Input: part model. Units: mm. Frame: model coordinates. Face numbers are marked on the shaded views. A direction names the side the tool comes from. Coordinates: 2 decimals unless noted, no trailing zeros. Write each loop counter-clockwise with the first axis right and the second up, starting at its lowest first coordinate (ties: lowest second). Pieces come first, ordered by that corner, then holes.
from build123d import *

# Parameters (mm, degrees)
F0_W      = 96
F0_H      = 12
F1_DEPTH  = 18
F3_DEPTH  = 10
F4_R      = 17
F5_R      = 6
F6_DEPTH  = 10.001
F7_W      = 14
F7_H      = 15
F8_DEPTH  = 25
F9_R      = 7
F10_DEPTH = 25
F11_R     = 5
F12_DEPTH = 12.001


with BuildPart() as f1:
    # F0 (on Front) → F1 (new body, symmetric)
    with BuildSketch(Plane.XZ):
        Rectangle(F0_W, F0_H)
    extrude(amount=F1_DEPTH, both=True)

    # F2 (on face) → F3 (join)
    with BuildSketch(Plane(origin=(0, 18, 0), x_dir=(-1, 0, 0), z_dir=(0, 1, 0))):
        Polygon((0, 37.958633), (-48, 6), (48, 6), align=None)
    extrude(amount=-F3_DEPTH)

    # F4
    f4_edges = [f1.edges().sort_by_distance(p)[0] for p in [
        (0, 13, 37.958633),
    ]]
    fillet(f4_edges, radius=F4_R)

    # F5 (on face) → F6 (cut, through all)
    with BuildSketch(Plane.XZ.offset(-8)):
        with Locations((0, 21)):
            Circle(F5_R)
    extrude(amount=-F6_DEPTH, mode=Mode.SUBTRACT)

    # F7 (on face) → F8 (cut)
    with BuildSketch(Plane.XY.offset(6)):
        with Locations((0, -10.5)):
            Rectangle(F7_W, F7_H)
        with Locations((0, -25.5)):
            Rectangle(F7_W, F7_H)
    extrude(amount=-F8_DEPTH, mode=Mode.SUBTRACT)

    # F9 (on face) → F10 (cut)
    with BuildSketch(Plane.XY.offset(6)):
        with Locations((0, -3)):
            Circle(F9_R)
    extrude(amount=-F10_DEPTH, mode=Mode.SUBTRACT)

    # F11 (on face) → F12 (cut, through all)
    with BuildSketch(Plane.XY.offset(6)):
        with Locations((36, -6)):
            Circle(F11_R)
        with Locations((-36, -6)):
            Circle(F11_R)
    extrude(amount=-F12_DEPTH, mode=Mode.SUBTRACT)


solid = f1.part
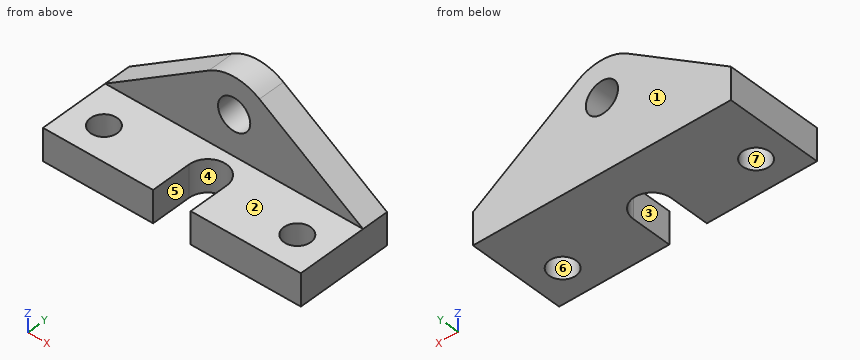
Item 1: Pull-direction query (Y, two-part tool) for the marked faces 4, 5, 6 and 7; classes: released by +Y, released by -Y, zero draft, split by the parting line, or undercut.
Item 2: Access query for the marked faces 1, 2 and 3. Directions: +Z, -Z, +X, -X, +Y, -Y. A direction counts if a zero-diameter tool reaches every point of the face in a straight line with its end or side. Return the directions, or none.
Item 3: Section query B-B, the plane x = 0. Return loops of the section in (y, z).
Item 4: Pin query (flat end, axial travel): pin 1 Ø14.5 at (x, z) = (-9.5, 16) entering from -Y; pin 2 Ø1.5 at (x, y) = (-26.5, 4) entering from +Z; pin 3 Ø10 at (y, z) = (14.5, 28) entering from +X. Return the tip coordinate at first contact, or that it passes through.
Item 5: Material intervals for line 1 (Y direction, x = -36, z = -2); line 2 (X direction, y = -3.5, z = 5); line 3 (Z direction, x = 35, y = -15), sorted ascending.
Item 6: Section query C-C, the plane z = 16. Return loops of the section in (x, y).
Item 7: Section query A-A, the plane y = -6. Return loops of the section in (x, z), then the cut area to 3 significant figures.
Item 8: Section query D-D, the plane x = 20.5. Return loops of the section in (y, z), then the cut area to 3 significant figures.
The answers:
1. face 4: released by -Y
1. face 5: zero draft
1. face 6: undercut
1. face 7: undercut
2. face 1: +Z, -Z, +X, -X, +Y
2. face 2: +Z, +X, -X, -Y
2. face 3: +Z, -Z, -Y
3. outline: (4, -6) - (18, -6) - (18, 15) - (8, 15) - (8, 6) - (4, 6) - close; (8, 27) - (18, 27) - (18, 34.54) - (8, 34.54) - close
4. pin 1: stops at y = 8
4. pin 2: stops at z = 6
4. pin 3: stops at x = 22.47
5. line 1: y = -18 to -11, -1 to 18
5. line 2: x = -48 to -40.33, -31.67 to -7, 7 to 31.67, 40.33 to 48
5. line 3: z = -6 to 6
6. outline: (-32.98, 8) - (-3.32, 8) - (-3.32, 18) - (-32.98, 18) - close; (3.32, 8) - (32.98, 8) - (32.98, 18) - (3.32, 18) - close
7. outline: (-48, -6) - (-41, -6) - (-41, 6) - (-48, 6) - close; (-31, -6) - (-7, -6) - (-7, 6) - (-31, 6) - close; (7, -6) - (31, -6) - (31, 6) - (7, 6) - close; (41, -6) - (48, -6) - (48, 6) - (41, 6) - close
7. area: 744 mm2
8. outline: (-18, -6) - (18, -6) - (18, 24.31) - (8, 24.31) - (8, 6) - (-18, 6) - close
8. area: 615 mm2
